Build history of the part. All positions in model axes, mm. A direction names the side the tool comes from. Coordinates: 2 decimals unless noted, no trailing zeros. Order: outer loops, then holes, each group sorted by start corner. A loop starts at its lowest first (then second) coordinate and runs counter-clockwise, first axis right, second up. Notation, with made-up numbers: (25.25, 5) - (78.25, 5) arc R25 cw to (78.25, 42) - close; hole circle Ø8 at (-40, 70.5). An arc over 180 degrees is marked (long way). Write each question's results on one line, items separated by ' | '.
from build123d import *

# Parameters (mm, degrees)
CROQUIS1_R              = 25.5
SALIENTE_EXTRUIR1_DEPTH = 10
CORTAR_EXTRUIR1_REACH   = 12
CROQUIS2_R              = 1.5


with BuildPart() as part:
    # Croquis1 → Saliente-Extruir1 (new body)
    with BuildSketch(Plane(origin=(0, 0, 0), x_dir=(1, 0, 0), z_dir=(0, 1, 0))):
        Polygon((40, -10), (50, -10), (50, 0), (-50, 0), (-50, -10), (-40, -10), (-25.121040683, -80), (-25.121040683, -110), (-7.121040683, -110), (-7.121040683, -85), (7.121040683, -85), (7.121040683, -110), (25.121040683, -110), (25.121040683, -80), align=None)
        with Locations((0, -52)):
            Circle(CROQUIS1_R, mode=Mode.SUBTRACT)
    extrude(amount=SALIENTE_EXTRUIR1_DEPTH)

    # Croquis2 → Cortar-Extruir1 (cut, up to next)
    with BuildSketch(Plane.XY.offset(10), mode=Mode.PRIVATE) as cortar_extruir1_sk1:
        with Locations((-45, 5)):
            Circle(CROQUIS2_R)
    cortar_extruir1_tool1 = extrude(cortar_extruir1_sk1.sketch, amount=-CORTAR_EXTRUIR1_REACH, mode=Mode.PRIVATE) & part.part
    add(cortar_extruir1_tool1.solids().sort_by_distance((-45, 5, 10))[0], mode=Mode.SUBTRACT)
    # Croquis2 → Cortar-Extruir1 (cut, up to next)
    with BuildSketch(Plane.XY.offset(10), mode=Mode.PRIVATE) as cortar_extruir1_sk2:
        with Locations((45, 5)):
            Circle(CROQUIS2_R)
    cortar_extruir1_tool2 = extrude(cortar_extruir1_sk2.sketch, amount=-CORTAR_EXTRUIR1_REACH, mode=Mode.PRIVATE) & part.part
    add(cortar_extruir1_tool2.solids().sort_by_distance((45, 5, 10))[0], mode=Mode.SUBTRACT)


solid = part.part
1. Band-saw the part on B-B on x = 0. Give the cut face in (y, z).
Solved:
outline: (0, 0) - (10, 0) - (10, 26.5) - (0, 26.5) - close; (0, 77.5) - (10, 77.5) - (10, 85) - (0, 85) - close
2. Probe line 1 (Z direction, x = -1, y = 2); line 2 (X direction, y = 5.75, z = 97.5); line 3 (Y direction, x = -45, z = 4.5). List the from-to ranges inside material, lowest first.
Solved:
line 1: z = 0 to 26.52, 77.48 to 85 | line 2: x = -25.12 to -7.12, 7.12 to 25.12 | line 3: y = 0 to 3.5, 6.5 to 10
3. Drop flat-ended pins along their axis: pin 1 Ø3 at (y, z) = (6.5, 94.5) entering from +X; pin 2 Ø3 at (x, y) = (2.5, 5.5) entering from +Z; pin 3 Ø3 at (y, z) = (3, 93) entering from -X. Give the stop position or say it passes through.
Solved:
pin 1: stops at x = 25.12 | pin 2: stops at z = 85 | pin 3: stops at x = -25.12
4. Band-saw the part on D-D on z = 21.5. Give the cut face in (x, y).
Solved:
outline: (-37.56, 0) - (37.56, 0) - (37.56, 10) - (-37.56, 10) - close
5. Band-saw the part on C-C on z = 99. Give the cut face in (x, y).
Solved:
outline: (-25.12, 0) - (-7.12, 0) - (-7.12, 10) - (-25.12, 10) - close; (7.12, 0) - (25.12, 0) - (25.12, 10) - (7.12, 10) - close
6. Band-saw the part on A-A on y = 5. Give the cut face in (x, z), then the cut area to 3 significant figures.
Solved:
outline: (-50, 0) - (-46.5, 0) - (-46.5, 10) - (-50, 10) - close; (-43.5, 0) - (43.5, 0) - (43.5, 10) - (40, 10) - (25.12, 80) - (25.12, 110) - (7.12, 110) - (7.12, 85) - (-7.12, 85) - (-7.12, 110) - (-25.12, 110) - (-25.12, 80) - (-40, 10) - (-43.5, 10) - close; (46.5, 0) - (50, 0) - (50, 10) - (46.5, 10) - close; hole circle Ø51 at (0, 52) | area: 4,610 mm2
7. Two-plate mould, pull along Y, no slides. Class faces 1 (the face through (-3.32, 4.93, 26.717)), 2 (the face through (22, 10, 30)), 3 (the face through (43.5, 5.07, 5.07)): +Y half, -Y half, draft (parallel to the pull), parting line (faces both ways), or undercut.
Solved:
face 1: draft | face 2: +Y half | face 3: undercut
8. Tool access for faces 4 (the face through (0, 5, 85)), 5 (the face through (-46.2, 3.8, 10)), 6 (the face through (43.8, 3.8, 10)): list every direction of +Z, -Z, +X, -X, +Y, -Y with a clear straight run to the whole face (end or side of a thin tool).
Solved:
face 4: +Z, +Y, -Y | face 5: +Z, -X, +Y, -Y | face 6: +Z, +X, +Y, -Y
